Source: CAD feature listing. Evaluate the final solid. Frame: model axes, mm. Face numbers are marked on the shaded views. A direction names the side the tool comes from. Round coordinates to 2 decimals unless told otherwise and drop trailing zeros. Loops run counter-clockwise (first coordinate to the right, second up) from the corner with the lowest first, then second, coordinate; pieces in that order, holes last.
(1) Section A-A, the plane x = 80.5. Return the cut outline in (y, z).
(2) Set-up query: the marked faces 1 and 2. Return all of +Z, -Z, +X, -X, +Y, -Y with unobstructed straight access to the full face (end or side cutting, diameter ignored); none if empty.
(3) Material intervals for probe 1 along X at (y, z) = (45.5, 27.5); probe 2 along X at (y, z) = (7, 33); probe 3 along X at (y, z) = (74, 16.5), sorted ascending.
(4) Section C-C, the plane y = 74. Return the cut outline in (x, z), plus the area to 3 significant figures.
(5) Section D-D, the plane z = 25. Return the cut outline in (x, y).
(6) Section B-B, the plane y = 25. Count the separate pieces of the cut face and the enclosed holes in it, plus the area to 3 significant figures.
(7) Mould query, pull axis Y, two halves, no side actions, for the marked faces 3, 4 and 5. Classes: pulls with the +Y half, pulls with the -Y half, needs draft (parallel to the pull), parting line crosses it, or undercut.
(8) First-contact query: pin 1 Ø2.5 at (y, z) = (44.5, 2) entering from -X; pin 2 Ø12 at (x, z) = (-69, 15) entering from +Y; pin 3 Ø2 at (y, z) = (30.5, 20.5) entering from -X. Flat tips, straight axial feed; report the tip coordinate or a pass-through.
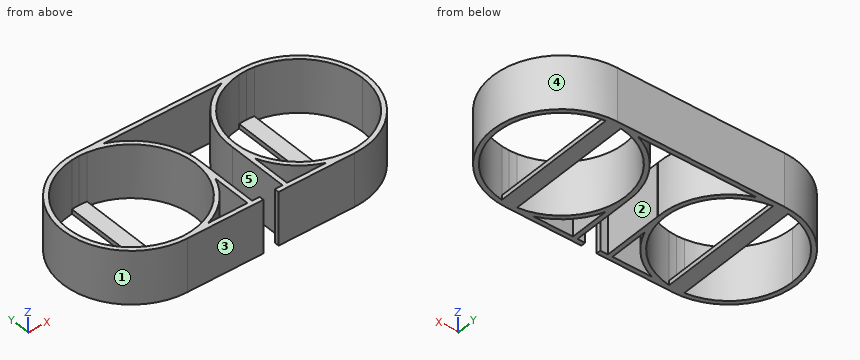
```python
from build123d import *

# Parameters (mm, degrees)
F0_W     = 5
F0_H     = 3
F1_DEPTH = 35
F2_DEPTH = 3


with BuildPart() as f1:
    # F0 (on Top) → F1 (new body)
    with BuildSketch(Plane.XY):
        with Locations((7.5, 1.5)):
            Rectangle(F0_W, F0_H)
        with BuildLine():
            Line((10, 3), (10, 0))
            Line((10, 0), (55, 0))
            ThreePointArc((55, 0), (46.7841616374, 0.7563563887), (38.8445055786, 3))
            Line((38.8445055786, 3), (13, 3))
            Line((13, 3), (10, 3))
        make_face()
        with BuildLine():
            Line((10, 43), (10, 3))
            Line((10, 3), (13, 3))
            Line((13, 3), (13, 28.8445055786))
            ThreePointArc((13, 28.8445055786), (10.9499068005, 35.8027564392), (10.044466414, 43))
            Line((10.044466414, 43), (10, 43))
        make_face()
        with BuildLine():
            ThreePointArc((38.8445055786, 3), (46.7841616374, 0.7563563887), (55, 0))
            Line((55, 0), (55, 3))
            Line((55, 3), (38.8445055786, 3))
        make_face()
        with BuildLine():
            Line((38.8445055786, 3), (55, 3))
            ThreePointArc((55, 3), (52.4955434529, 3.074736764), (50, 3.298681076))
            ThreePointArc((50, 3.298681076), (13, 45), (50, 86.701318924))
            ThreePointArc((50, 86.701318924), (52.4955434529, 86.925263236), (55, 87))
            Line((55, 87), (38.8445055786, 87))
            ThreePointArc((38.8445055786, 87), (17.3484470967, 69.6446863232), (10.044466414, 43))
            Line((10.044466414, 43), (13, 43))
            Line((13, 43), (13, 28.8445055786))
            ThreePointArc((13, 28.8445055786), (23.1801948466, 13.1801948466), (38.8445055786, 3))
        make_face()
        with BuildLine():
            Line((55, 3), (55, 0))
            ThreePointArc((55, 0), (86.8198051534, 13.1801948466), (100, 45))
            ThreePointArc((100, 45), (86.8198051534, 76.8198051534), (55, 90))
            Line((55, 90), (55, 87))
            ThreePointArc((55, 87), (57.5044565471, 86.925263236), (60, 86.701318924))
            ThreePointArc((60, 86.701318924), (86.4165561448, 72.8747197295), (97, 45))
            ThreePointArc((97, 45), (86.4165561448, 17.1252802705), (60, 3.298681076))
            ThreePointArc((60, 3.298681076), (57.5044565471, 3.074736764), (55, 3))
        make_face()
        with BuildLine():
            Line((55, 87), (55, 90))
            ThreePointArc((55, 90), (46.7841616374, 89.2436436113), (38.8445055786, 87))
            Line((38.8445055786, 87), (55, 87))
        make_face()
        with BuildLine():
            ThreePointArc((38.8445055786, 87), (46.7841616374, 89.2436436113), (55, 90))
            Line((55, 90), (0, 90))
            Line((0, 90), (0, 87))
            Line((0, 87), (38.8445055786, 87))
        make_face()
        with BuildLine():
            ThreePointArc((10.044466414, 43), (10.9499068005, 35.8027564392), (13, 28.8445055786))
            Line((13, 28.8445055786), (13, 43))
            Line((13, 43), (10.044466414, 43))
        make_face()
    extrude(amount=F1_DEPTH)

    # F0 (on Top) → F2 (join)
    with BuildSketch(Plane.XY):
        with BuildLine():
            Line((50, 45), (55, 45))
            Line((55, 45), (55, 87))
            ThreePointArc((55, 87), (52.4955434529, 86.925263236), (50, 86.701318924))
            Line((50, 86.701318924), (50, 45))
        make_face()
        with BuildLine():
            Line((55, 87), (55, 45))
            Line((55, 45), (60, 45))
            Line((60, 45), (60, 86.701318924))
            ThreePointArc((60, 86.701318924), (57.5044565471, 86.925263236), (55, 87))
        make_face()
        with BuildLine():
            ThreePointArc((50, 3.298681076), (52.4955434529, 3.074736764), (55, 3))
            Line((55, 3), (55, 45))
            Line((55, 45), (50, 45))
            Line((50, 45), (50, 3.298681076))
        make_face()
        with BuildLine():
            Line((55, 45), (55, 3))
            ThreePointArc((55, 3), (57.5044565471, 3.074736764), (60, 3.298681076))
            Line((60, 3.298681076), (60, 45))
            Line((60, 45), (55, 45))
        make_face()
    extrude(amount=F2_DEPTH)

    # F3: F1 across plane


with BuildPart() as f1_1:
    add(f1.part)
    add(f1.part.mirror(Plane.YZ))


solid = f1_1.part
```
Output values:
1. outline: (7.92, 0) - (11.63, 0) - (11.63, 35) - (7.92, 35) - close; (78.37, 0) - (82.08, 0) - (82.08, 35) - (78.37, 35) - close
2. face 1: +Z, -Z, -X
2. face 2: +Z, -Z
3. probe 1: x = -100 to -97, -13 to -10, 10 to 13, 97 to 100
3. probe 2: x = -79.1 to -72.89, -37.11 to -30.9, -13 to -10, 10 to 13, 30.9 to 37.11, 72.89 to 79.1
3. probe 3: x = -89.41 to -85.38, -24.62 to -20.59, 20.59 to 24.62, 85.38 to 89.41
4. outline: (-89.41, 0) - (-85.38, 0) - (-85.38, 35) - (-89.41, 35) - close; (-60, 0) - (-50, 0) - (-50, 3) - (-60, 3) - close; (-24.62, 0) - (-20.59, 0) - (-20.59, 35) - (-24.62, 35) - close; (20.59, 0) - (24.62, 0) - (24.62, 35) - (20.59, 35) - close; (50, 0) - (60, 0) - (60, 3) - (50, 3) - close; (85.38, 0) - (89.41, 0) - (89.41, 35) - (85.38, 35) - close
4. area: 624 mm2
5. outline: (-55, 0) - (-5, 0) - (-5, 3) - (-10, 3) - (-10, 43) - (-10.04, 43) arc R45 ccw to (-38.84, 87) - (38.84, 87) arc R45 ccw to (10.04, 43) - (10, 43) - (10, 3) - (5, 3) - (5, 0) - (55, 0) arc R45 ccw to (55, 90) - (-55, 90) arc R45 ccw to start; hole circle Ø84 at (-55, 45); hole (-38.84, 3) - (-13, 3) - (-13, 28.84) arc R45 cw to start; hole (13, 3) - (38.84, 3) arc R45 cw to (13, 28.84) - close; hole circle Ø84 at (55, 45)
6. separate pieces: 8
6. enclosed holes: 0
6. area: 743 mm2
7. face 3: pulls with the -Y half
7. face 4: parting line crosses it
7. face 5: undercut
8. pin 1: stops at x = -100
8. pin 2: stops at y = 89.28
8. pin 3: stops at x = -97.93
